from build123d import *

# Parameters (mm, degrees)
SKETCH1_R             = 27.8
BOSS_EXTRUDE1_DEPTH   = 4.8
CHAMFER1_SIZE         = 2
CUT_EXTRUDE1_START    = -3.56
CUT_EXTRUDE1_DEPTH    = 3.56
M3X0_5_TAPPED_HOLE1_D = 2.5
SKETCH7_R             = 4
CUT_EXTRUDE2_DEPTH    = 40.607070076
SKETCH8_R             = 6.5
CUT_EXTRUDE3_DEPTH    = 1.2
M3X0_5_TAPPED_HOLE2_D = 2.5


with BuildPart() as part:
    # Sketch1 → Boss-Extrude1 (new body)
    with BuildSketch(Plane.XY):
        Circle(SKETCH1_R)
    extrude(amount=BOSS_EXTRUDE1_DEPTH)

    # Chamfer1
    chamfer1_edges = [part.edges().sort_by_distance(p)[0] for p in [
        (-27.8, 0, 4.8),
    ]]
    chamfer(chamfer1_edges, length=CHAMFER1_SIZE)

    # Sketch2 → Cut-Extrude1 (cut)
    with BuildSketch(Plane.XY.offset(4.8).offset(CUT_EXTRUDE1_START)):
        with BuildLine():
            Line((-3.02, 27.635477199), (-3.02, 24.78))
            ThreePointArc((-3.02, 24.78), (0, 21.76), (3.02, 24.78))
            Line((3.02, 24.78), (3.02, 27.635477199))
            ThreePointArc((3.02, 27.635477199), (0, 27.8), (-3.02, 27.635477199))
        make_face()
        with BuildLine():
            Line((22.4230253, 16.433135319), (19.950109506, 15.005396719))
            ThreePointArc((19.950109506, 15.005396719), (18.844712786, 10.88), (22.970109506, 9.774603281))
            Line((22.970109506, 9.774603281), (25.4430253, 11.20234188))
            ThreePointArc((25.4430253, 11.20234188), (24.075506225, 13.9), (22.4230253, 16.433135319))
        make_face()
        with BuildLine():
            Line((25.4430253, -11.20234188), (22.970109506, -9.774603281))
            ThreePointArc((22.970109506, -9.774603281), (18.844712786, -10.88), (19.950109506, -15.005396719))
            Line((19.950109506, -15.005396719), (22.4230253, -16.433135319))
            ThreePointArc((22.4230253, -16.433135319), (24.075506225, -13.9), (25.4430253, -11.20234188))
        make_face()
        with BuildLine():
            Line((3.02, -27.635477199), (3.02, -24.78))
            ThreePointArc((3.02, -24.78), (0, -21.76), (-3.02, -24.78))
            Line((-3.02, -24.78), (-3.02, -27.635477199))
            ThreePointArc((-3.02, -27.635477199), (0, -27.8), (3.02, -27.635477199))
        make_face()
        with BuildLine():
            Line((-22.4230253, -16.433135319), (-19.950109506, -15.005396719))
            ThreePointArc((-19.950109506, -15.005396719), (-18.844712786, -10.88), (-22.970109506, -9.774603281))
            Line((-22.970109506, -9.774603281), (-25.4430253, -11.20234188))
            ThreePointArc((-25.4430253, -11.20234188), (-24.075506225, -13.9), (-22.4230253, -16.433135319))
        make_face()
        with BuildLine():
            Line((-25.4430253, 11.20234188), (-22.970109506, 9.774603281))
            ThreePointArc((-22.970109506, 9.774603281), (-18.844712786, 10.88), (-19.950109506, 15.005396719))
            Line((-19.950109506, 15.005396719), (-22.4230253, 16.433135319))
            ThreePointArc((-22.4230253, 16.433135319), (-24.075506225, 13.9), (-25.4430253, 11.20234188))
        make_face()
        with BuildLine():
            ThreePointArc((-8.990760958, 18.077325331), (-7.097001538, 19.802867047), (-8.218352654, 22.106427471))
            Line((-8.218352654, 22.106427471), (-10.434772365, 23.595667519))
            Line((-10.434772365, 23.595667519), (-11.326579695, 26.037938541))
            ThreePointArc((-11.326579695, 26.037938541), (-14.197408663, 24.590633141), (-16.886226391, 22.828075024))
            Line((-16.886226391, 22.828075024), (-15.217061308, 20.834611711))
            Line((-15.217061308, 20.834611711), (-15.035551449, 18.170515911))
            ThreePointArc((-15.035551449, 18.170515911), (-13.601285161, 16.047617146), (-11.16004249, 16.824890055))
            ThreePointArc((-11.16004249, 16.824890055), (-10.211194098, 17.686306984), (-8.990760958, 18.077325331))
        make_face()
        with BuildLine():
            ThreePointArc((8.990760958, -18.077325331), (7.097001538, -19.802867047), (8.218352654, -22.106427471))
            Line((8.218352654, -22.106427471), (10.434772365, -23.595667519))
            Line((10.434772365, -23.595667519), (11.326579695, -26.037938541))
            ThreePointArc((11.326579695, -26.037938541), (14.197408663, -24.590633141), (16.886226391, -22.828075024))
            Line((16.886226391, -22.828075024), (15.217061308, -20.834611711))
            Line((15.217061308, -20.834611711), (15.035551449, -18.170515911))
            ThreePointArc((15.035551449, -18.170515911), (13.601285161, -16.047617146), (11.16004249, -16.824890055))
            ThreePointArc((11.16004249, -16.824890055), (10.211194098, -17.686306984), (8.990760958, -18.077325331))
        make_face()
        with BuildLine():
            ThreePointArc((9.592925481, 14.639879042), (10.072666849, 13.587453118), (11.224576406, 13.691647537))
            ThreePointArc((11.224576406, 13.691647537), (14.666706062, 17.996812228), (16.27190214, 23.26995599))
            ThreePointArc((16.27190214, 23.26995599), (13.319162757, 25.077191918), (10.168440088, 26.511666813))
            ThreePointArc((10.168440088, 26.511666813), (10.298392669, 20.555523396), (9.592925481, 14.639879042))
        make_face()
        with BuildLine():
            ThreePointArc((28.288324102, 2.456902626), (22.919049608, 3.703333926), (17.46960279, 2.874944546))
            ThreePointArc((17.46960279, 2.874944546), (16.803412997, 1.929458816), (17.474969899, 0.987777643))
            ThreePointArc((17.474969899, 0.987777643), (22.950801784, -1.359092028), (28.043997001, -4.449705973))
            ThreePointArc((28.043997001, -4.449705973), (28.377066635, -1.003862654), (28.288324102, 2.456902626))
        make_face()
        with BuildLine():
            ThreePointArc((-28.288324102, -2.456902626), (-22.919049608, -3.703333926), (-17.46960279, -2.874944546))
            ThreePointArc((-17.46960279, -2.874944546), (-16.803412997, -1.929458816), (-17.474969899, -0.987777643))
            ThreePointArc((-17.474969899, -0.987777643), (-22.950801784, 1.359092028), (-28.043997001, 4.449705973))
            ThreePointArc((-28.043997001, 4.449705973), (-28.377066635, 1.003862654), (-28.288324102, -2.456902626))
        make_face()
        with BuildLine():
            ThreePointArc((-10.168440088, -26.511666813), (-10.298392669, -20.555523396), (-9.592925481, -14.639879042))
            ThreePointArc((-9.592925481, -14.639879042), (-10.072666849, -13.587453118), (-11.224576406, -13.691647537))
            ThreePointArc((-11.224576406, -13.691647537), (-14.666706062, -17.996812228), (-16.27190214, -23.26995599))
            ThreePointArc((-16.27190214, -23.26995599), (-13.319162757, -25.077191918), (-10.168440088, -26.511666813))
        make_face()
    extrude(amount=CUT_EXTRUDE1_DEPTH, mode=Mode.SUBTRACT)

    # M3x0.5 Tapped Hole1 (through all)
    with Locations(Plane.XY.offset(4.8)):
        with Locations((0, 15), (12.990881057, 7.500866025), (12.991881057, -7.499133975), (7.501866025, -12.989881057), (0.002, -15), (-12.988881057, -7.500866025), (-12.989881057, 7.499133975), (-7.499866025, 12.989881057)):
            Hole(M3X0_5_TAPPED_HOLE1_D / 2)

    # Sketch7 → Cut-Extrude2 (cut, through all)
    with BuildSketch(Plane.XY.offset(4.8)):
        Circle(SKETCH7_R)
    extrude(amount=-CUT_EXTRUDE2_DEPTH, mode=Mode.SUBTRACT)

    # Sketch8 → Cut-Extrude3 (cut)
    with BuildSketch(Plane.XY.offset(4.8)):
        Circle(SKETCH8_R)
    extrude(amount=-CUT_EXTRUDE3_DEPTH, mode=Mode.SUBTRACT)

    # M3x0.5 Tapped Hole2 (through all)
    with Locations(Plane.XY.offset(4.8)):
        with Locations((0, 24.78), (21.460109506, 12.39), (21.460109506, -12.39), (0, -24.78), (-21.460109506, -12.39), (-21.460109506, 12.39), (0, 0)):
            Hole(M3X0_5_TAPPED_HOLE2_D / 2)


solid = part.part
Read the model definition and answer for the solid it produces. Units are mm, in the model's axes. A direction names the side the tool comes from. Give positions to 0.01 mm unless a question says otherwise; leave off trailing zeros. Write each loop counter-clockwise with the first axis right and the second up, starting at its lowest first coordinate (ties: lowest second). Pieces come first, ordered by that corner, then holes. Notation, with made-up numbers: (-19.5, 17.5) - (-11.5, 17.5) arc R20 ccw to (-11.5, 41.5) - close; hole circle Ø4 at (-37.75, 57.25). An arc over 180 degrees is marked (long way). Return JSON: item names as keys, results as strings.
Q1. Consider line 1 along Y through (x, z) = (0, 2.45); line 2 along Y through (x, z) = (0, 0.3); line 3 along X through (y, z) = (-11, 1.7). Determine where each line is inside the solid, lowest interval first. Write a range as [from, to].
Reply:
{"line 1": "[-21.76, -16.25], [-13.75, -4], [4, 13.75], [16.25, 21.76]", "line 2": "[-27.8, -26.03], [-23.53, -16.25], [-13.75, -4], [4, 13.75], [16.25, 23.53], [26.03, 27.8]", "line 3": "[-25.53, -25.09], [-18.78, 18.78], [25.09, 25.53]"}
Q2. For a pull along X with two mould halves and no side action, classify faces 6 (the face through (-18.9, 19, 3.8)), 7 (the face through (23, -13, 1.24)), 8 (the face through (6.95, 25.87, 3.81)), 9 (the face through (-23.914, -10.32, 2.6)) as released by +X, released by -X, zero draft, split by the parting line, or undercut.
Reply:
{"face 6": "released by -X", "face 7": "undercut", "face 8": "released by +X", "face 9": "undercut"}
Q3. A cutting plane is placed at A-A, the plane x = 0. Count the separate pieces of the cut face and the enclosed holes in it, and give its area (3 significant figures).
Reply:
{"separate pieces": "6", "enclosed holes": "0", "area": "149 mm²"}
Q4. For faces 1 (the face through (-7.105, 19.765, 2.995)), 2 (the face through (14.471, 17.637, 2.995)), 3 (the face through (20.89, -15.55, 2.6)), 4 (the face through (23.95, -10.34, 2.6)), 5 (the face through (-10.697, 24.315, 2.6)), determine the directions among +Z, -Z, +X, -X, +Y, -Y from which every point of the face is accessible in a straight line to the end or side of a thin tool.
Reply:
{"face 1": "+Z", "face 2": "+Z, +Y", "face 3": "+Z, +X", "face 4": "+Z, -Y", "face 5": "+Z, -X"}
Q5. A cutting plane is placed at B-B, the plane y = 0. Determine the outline of the cut face in (x, z), and give its area (3 significant figures).
Reply:
{"outline": "(-27.8, 0) - (-4, 0) - (-4, 3.6) - (-6.5, 3.6) - (-6.5, 4.8) - (-20.04, 4.8) - (-20.04, 1.24) - (-27.8, 1.24) - close; (4, 0) - (27.8, 0) - (27.8, 1.24) - (20.04, 1.24) - (20.04, 4.8) - (6.5, 4.8) - (6.5, 3.6) - (4, 3.6) - close", "area": "167 mm²"}
Q6. Given P1, Ø1.4, axis at y = 25.5, z = 2.5, coming from the -X side; P2, Ø2, axis at x = -7.5, y = 12.99, coming from the +Z side (1 decimal); P3, Ø1.5, axis at x = 21, z = 3, coming from the +Y side; P4, Ø1, axis at y = 2.5, z = 2.5, coming from the +X side, each flat-ended and moving along its own axis, determine where each tip first touches the part or whether it passes through.
Reply:
{"P1": "x = -11.12", "P2": "through", "P3": "y = 19.02", "P4": "x = 27.67"}
